```python
from build123d import *

# Parameters (mm, degrees)
SKETCH1_W               = 114.045996948
SKETCH1_H               = 72.771003052
SKETCH1_W_2             = 108.965996948
SKETCH1_H_2             = 67.691003052
BOSS_EXTRUDE1_DEPTH     = 5.3848
SKETCH2_W               = 114.045996948
SKETCH2_H               = 72.771003052
BOSS_EXTRUDE2_DEPTH     = 2.54
SKETCH3_W               = 9.64565
SKETCH3_H               = 9.645653052
BOSS_EXTRUDE3_DEPTH     = 3.81
CUT_EXTRUDE1_DEPTH      = 132.233284578
CUT_EXTRUDE1_DEPTH_BACK = 76.2
SKETCH4_R               = 2.1499957
SKETCH5_R               = 3.8735
CUT_EXTRUDE2_DEPTH      = 2.54
BOSS_EXTRUDE4_DEPTH     = 1.27
BOSS_EXTRUDE5_DEPTH     = 1.27
FILLET1_R               = 1.27


with BuildPart() as part:
    # Sketch1 → Boss-Extrude1 (new body)
    with BuildSketch(Plane(origin=(0, 0, 0), x_dir=(1, 0, 0), z_dir=(0, 1, 0))):
        with Locations((53.974998474, 33.337501526)):
            Rectangle(SKETCH1_W, SKETCH1_H)
        with Locations((53.974998474, 33.337501526)):
            Rectangle(SKETCH1_W_2, SKETCH1_H_2, mode=Mode.SUBTRACT)
    extrude(amount=BOSS_EXTRUDE1_DEPTH)

    # Sketch2 → Boss-Extrude2 (add)
    with BuildSketch(Plane.XZ):
        with Locations((53.974998474, -33.337501526)):
            Rectangle(SKETCH2_W, SKETCH2_H)
    extrude(amount=BOSS_EXTRUDE2_DEPTH)

    # Sketch3 → Boss-Extrude3 (add)
    with BuildSketch(Plane(origin=(0, 0, 0), x_dir=(1, 0, 0), z_dir=(0, 1, 0))):
        with Locations((4.314825, 62.360176526)):
            Rectangle(SKETCH3_W, SKETCH3_H)
        with Locations((103.635171948, 62.360176526)):
            Rectangle(SKETCH3_W, SKETCH3_H)
        with Locations((103.635171948, 4.314826526)):
            Rectangle(SKETCH3_W, SKETCH3_H)
        with Locations((4.314825, 4.314826526)):
            Rectangle(SKETCH3_W, SKETCH3_H)
    extrude(amount=BOSS_EXTRUDE3_DEPTH)

    # Sketch4 → Cut-Extrude1 (cut, two sides: drawn at the far end of the back side and taken through both)
    with BuildSketch(Plane(origin=(0, 3.81, 0), x_dir=(1, 0, 0), z_dir=(0, 1, 0)).offset(-CUT_EXTRUDE1_DEPTH_BACK)):
        with Locations(Location((5.715, 60.96, 0), (0, 0, 90))):
            Circle(SKETCH4_R)
        with Locations(Location((5.715, 5.715, 0), (0, 0, 90))):
            Circle(SKETCH4_R)
        with Locations(Location((102.235, 5.715, 0), (0, 0, 90))):
            Circle(SKETCH4_R)
        with Locations(Location((102.235, 60.96, 0), (0, 0, 90))):
            Circle(SKETCH4_R)
    extrude(amount=CUT_EXTRUDE1_DEPTH + CUT_EXTRUDE1_DEPTH_BACK, mode=Mode.SUBTRACT)

    # Sketch5 → Cut-Extrude2 (cut)
    with BuildSketch(Plane.XZ.offset(2.54)):
        with Locations(Location((5.715, -60.96, 0), (0, 0, 270))):
            Circle(SKETCH5_R)
        with Locations(Location((5.715, -5.715, 0), (0, 0, 270))):
            Circle(SKETCH5_R)
        with Locations(Location((102.235, -60.96, 0), (0, 0, 270))):
            Circle(SKETCH5_R)
        with Locations(Location((102.235, -5.715, 0), (0, 0, 270))):
            Circle(SKETCH5_R)
    extrude(amount=-CUT_EXTRUDE2_DEPTH, mode=Mode.SUBTRACT)

    # Sketch6 → Boss-Extrude4 (add)
    with BuildSketch(Plane(origin=(0, 0, 0), x_dir=(1, 0, 0), z_dir=(0, 1, 0))):
        Polygon((9.13765, 67.183003052), (98.812346948, 67.183003052), (98.812346948, 57.53735), (108.457996948, 57.53735), (108.457996948, 9.137653052), (98.812346948, 9.137653052), (98.812346948, -0.508), (9.13765, -0.508), (9.13765, 9.137653052), (-0.508, 9.137653052), (-0.508, 57.53735), (9.13765, 57.53735), align=None)
    extrude(amount=BOSS_EXTRUDE4_DEPTH)

    # Sketch7 → Boss-Extrude5 (add)
    with BuildSketch(Plane(origin=(0, 5.3848, 0), x_dir=(1, 0, 0), z_dir=(0, 1, 0))):
        Polygon((-0.508, 67.183003052), (108.457996948, 67.183003052), (108.457996948, -0.508), (84.272696176, -0.508), (84.272696176, -1.524), (109.473996948, -1.524), (109.473996948, 68.199003052), (-1.524, 68.199003052), (-1.524, 41.825543933), (-0.508, 41.825543933), align=None)
        Polygon((-0.508, -0.508), (-0.508, 24.809543933), (-1.524, 24.809543933), (-1.524, -1.524), (67.256696176, -1.524), (67.256696176, -0.508), align=None)
    extrude(amount=BOSS_EXTRUDE5_DEPTH)

    # Fillet1
    fillet1_edges = [part.edges().sort_by_distance(p)[0] for p in [
        (110.997996948, -2.54, -33.337501526),
        (53.974998474, -2.54, 3.048),
        (-3.048, -2.54, -33.337501526),
        (53.974998474, -2.54, -69.723003052),
        (-3.048, 1.4224, -69.723003052),
        (110.997996948, 1.4224, -69.723003052),
        (110.997996948, 1.4224, 3.048),
        (-3.048, 1.4224, 3.048),
    ]]
    fillet(fillet1_edges, radius=FILLET1_R)


solid = part.part
```
Work out the finished part from the listing and answer in its coordinate system (mm). A direction names the side the tool comes from. Give positions to 0.01 mm unless a question says otherwise; leave off trailing zeros. Loops run counter-clockwise (first coordinate to the right, second up) from the corner with the lowest first, then second, coordinate; pieces in that order, holes last. Notation, with made-up numbers: (30, 34.5) -> (76, 34.5) arc R10 ccw to (76, 39.5) -> close; hole circle Ø4 at (24, 56). An arc over 180 degrees is marked (long way). Use CSV: the item, a comma, the result in double quotes.
1. The mould has two halves that part along Z. Classify faces 4 (the flat face through (53, 2, 3.048)), 5 (the flat face through (-3.048, 2, -34)), 6 (the cylindrical face through (104.334, 1.878, -5.249)), 7 (the flat face through (53, 2, -69.723)): +Z half, -Z half, draft (parallel to the pull), parting line (faces both ways), or undercut.
Found:
face 4,"+Z half"
face 5,"draft"
face 6,"undercut"
face 7,"-Z half"
2. The part is cut by section A-A (z = -60.96). State how many separate pieces and enclosed holes the cut face has, then the cut area to 3 significant figures.
Found:
separate pieces,"3"
enclosed holes,"0"
area,"434 mm^2"
3. The part is cut by section D-D (x = 30.5). Write down the section's boundary in (y, z).
Found:
outline,"(-2.54, -68.45) arc R1.27 ccw to (-1.27, -69.72) -> (5.38, -69.72) -> (5.38, -68.2) -> (6.65, -68.2) -> (6.65, -67.18) -> (1.27, -67.18) -> (1.27, 0.51) -> (6.65, 0.51) -> (6.65, 1.52) -> (5.38, 1.52) -> (5.38, 3.05) -> (-1.27, 3.05) arc R1.27 ccw to (-2.54, 1.78) -> close"
4. The part is cut by section B-B (x = 74). Write down the section's boundary in (y, z).
Found:
outline,"(-2.54, -68.45) arc R1.27 ccw to (-1.27, -69.72) -> (5.38, -69.72) -> (5.38, -68.2) -> (6.65, -68.2) -> (6.65, -67.18) -> (1.27, -67.18) -> (1.27, 0.51) -> (5.38, 0.51) -> (5.38, 3.05) -> (-1.27, 3.05) arc R1.27 ccw to (-2.54, 1.78) -> close"
5. The part is cut by section C-C (z = -44). Write down the section's boundary in (x, y).
Found:
outline,"(-3.05, -1.27) arc R1.27 ccw to (-1.78, -2.54) -> (109.73, -2.54) arc R1.27 ccw to (111, -1.27) -> (111, 5.38) -> (109.47, 5.38) -> (109.47, 6.65) -> (108.46, 6.65) -> (108.46, 1.27) -> (-0.51, 1.27) -> (-0.51, 6.65) -> (-1.52, 6.65) -> (-1.52, 5.38) -> (-3.05, 5.38) -> close"
6. Flat-ended cylindrical pins translate along their axes: pin 1 Ø1.1 at (x, y) = (-1, 6.5) entering from -Z; pin 2 Ø0.6 at (y, z) = (6, -53.5) entering from -X; pin 3 Ø0.5 at (y, z) = (6.5, 1) entering from +X. Find the tip coordinate at first contact, or state that the pin passes through.
Found:
pin 1,"z = -68.2"
pin 2,"x = -1.52"
pin 3,"x = 109.47"
7. A tool of negligible diameter and unlimited length cuts with its end or side. For faces 1 (the cylindrical face through (8.98, -1.29, -7.8)), 2 (the cylindrical face through (5.07, 1.88, -63.01)), 3 (the flat face through (55, 4, 0.508)), from which of +Z, -Z, +X, -X, +Y, -Y can it reach the whole face along a straight path? Write none if from no direction.
Found:
face 1,"-Y"
face 2,"+Y, -Y"
face 3,"+Y"
8. Straight lines are drawn through the part: line 1 (X direction, y = -1.4, z = -60.96); line 2 (X direction, y = 1.3, z = -60.96) (3 decimals); line 3 (Z direction, x = 54, y = 2). For each, find the intervals that lie inside material, in ascending order.
Found:
line 1,"-3.04 to 1.84, 9.59 to 98.36, 106.11 to 110.99"
line 2,"-3.048 to 3.565, 7.865 to 9.138, 98.812 to 100.085, 104.385 to 110.998"
line 3,"-69.72 to -67.18, 0.51 to 3.05"
